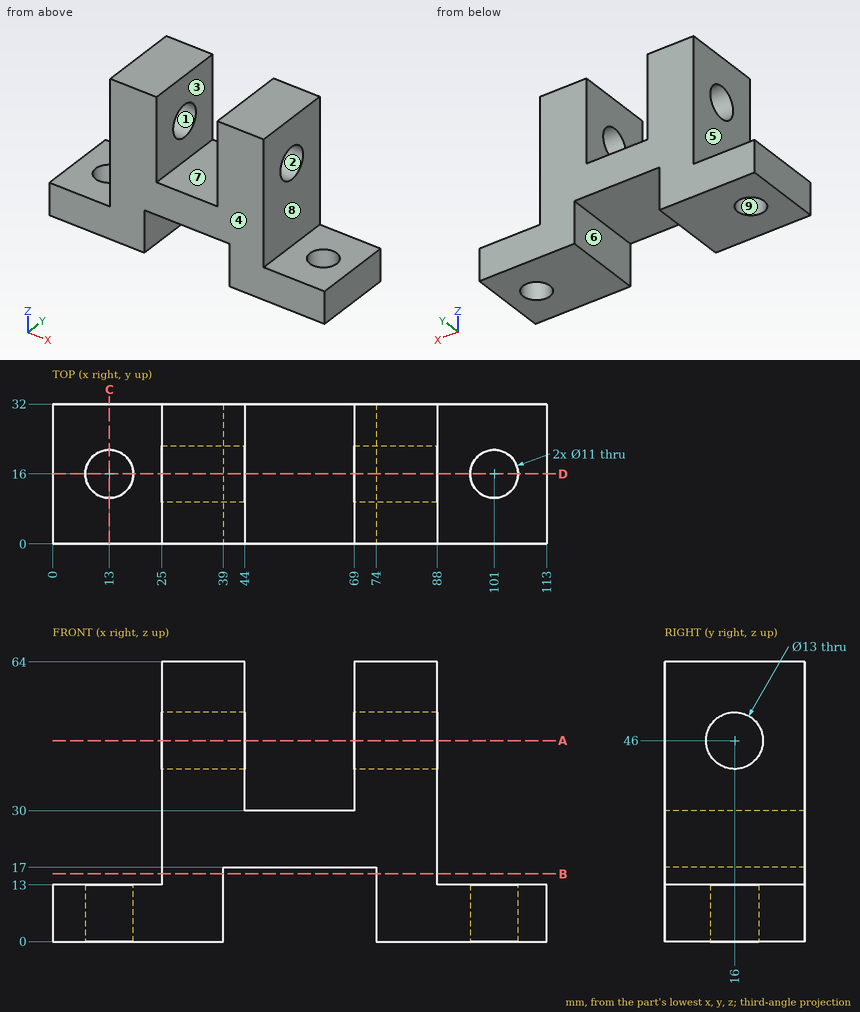
Geometry check sheet. Reference: drawing and pictorial views, mm from the part's lowest x, y, z. A direction names the side the tool comes from. Coordinates: 2 decimals unless noted, no trailing zeros. Write each loop counter-clockwise with the first axis right and the second up, starting at its lowest first coordinate (ties: lowest second). Pieces come first, ordered by that corner, then holes. Notation, with made-up numbers: M -26.75,17 L 0.25,17 A24 cw 0.25,28 Z; hole C -12.5,21 d10. An arc over 180 degrees is marked long. Use one line per item in the form item = value.
Item 1: Sectioned sample at B-B, the plane z = 15.5. Record the cut outline in (x, y), and give its area (3 significant figures).
Answer below:
outline = M 25,0 L 39,0 L 39,32 L 25,32 Z; M 74,0 L 88,0 L 88,32 L 74,32 Z
area = 896 mm^2
Item 2: Set-up check for the marked faces 5, 6, 7, 8 and 9: record each of +Z, -Z, +X, -X, +Y, -Y from which the full face is reachable in a straight line by a thin tool's end or side.
Answer below:
face_5 = +Z, -X, +Y, -Y
face_6 = -Z, +Y, -Y
face_7 = +Z, +Y, -Y
face_8 = +Z, +X, +Y, -Y
face_9 = +Z, -Z
Item 3: Release check for a two-part mould opening along Y. For the marked faces 1, 2, 3 and 4 record: pulls with the +Y half, pulls with the -Y half, needs draft (parallel to the pull), parting line crosses it, or undercut.
Answer below:
face_1 = undercut
face_2 = undercut
face_3 = needs draft
face_4 = pulls with the -Y half
Item 4: Gauge pin test, flat ends, axial feed: pin 1 Ø16 at (y, z) = (14.5, 44) entering from +X; pin 2 Ø9.5 at (y, z) = (23, 41.5) entering from -X; pin 3 Ø10.5 at (y, z) = (16, 46) entering from +X; pin 4 Ø12.5 at (x, y) = (7.5, 11.5) entering from +Z. Record the tip position at first contact, or that the pin passes through.
Answer below:
pin_1 = 88
pin_2 = 25
pin_3 = through
pin_4 = 13
Item 5: Sectioned sample at A-A, the plane z = 46. Record the cut outline in (x, y), and give its area (3 significant figures).
Answer below:
outline = M 25,0 L 44,0 L 44,9.5 L 25,9.5 Z; M 25,22.5 L 44,22.5 L 44,32 L 25,32 Z; M 69,0 L 88,0 L 88,9.5 L 69,9.5 Z; M 69,22.5 L 88,22.5 L 88,32 L 69,32 Z
area = 722 mm^2
Item 6: Material ranges on L1, parallel to X at y = 16, z = 10.5; L2, parallel to X at y = 22.5, z = 33; L3, parallel to Y at x = 83, z = 45.5, recorded low to high. Write a range as from..to.
Answer below:
L1 = 0..7.5, 18.5..39, 74..95.5, 106.5..113
L2 = 25..44, 69..88
L3 = 0..9.52, 22.48..32
Item 7: Sectioned sample at D-D, the plane y = 16. State how many separate pieces and enclosed holes the cut face has, and give its area (3 significant figures).
Answer below:
separate_pieces = 5
enclosed_holes = 0
area = 2,460 mm^2
Item 8: Sectioned sample at C-C, the plane x = 13. Record the cut outline in (y, z).
Answer below:
outline = M 0,0 L 10.5,0 L 10.5,13 L 0,13 Z; M 21.5,0 L 32,0 L 32,13 L 21.5,13 Z
